Check sheet for the modelled part. Datum: model origin and axes. Units: mm. A direction names the side the tool comes from. Round coordinates to 2 decimals unless told otherwise and drop trailing zeros. Order: outer loops, then holes, each group sorted by start corner. A loop starts at its lowest first (then second) coordinate and runs counter-clockwise, first axis right, second up. Notation, with made-up numbers: (5, -37.5) -> (37, -37.5) arc R22 ccw to (37, -22.5) -> close; hole circle Ø10 at (86, -26). An arc over 180 degrees is marked (long way). Answer in a Markdown table with one row per item.
from build123d import *

# Parameters (mm, degrees)
CUT_EXTRUDE_1_DEPTH = 4
FILLET_1_R          = 0.3
SKETCH_3_R          = 3
CUT_EXTRUDE_2_DEPTH = 25


with BuildPart() as part:
    # Эскиз1 → Повернуть1 (revolve)
    with BuildSketch(Plane.XY, mode=Mode.PRIVATE) as revolve_1_sk:
        with BuildLine():
            Line((0, 157), (0, 0))
            Line((0, 0), (23, 0))
            Line((23, 0), (23, 3.5))
            Line((23, 3.5), (14, 3.5))
            Line((14, 3.5), (14, 5.5))
            Line((14, 5.5), (15, 5.5))
            Line((15, 5.5), (15, 30.5))
            Line((15, 30.5), (13.5, 30.5))
            ThreePointArc((13.5, 30.5), (12.792893219, 30.792893219), (12.5, 31.5))
            Line((12.5, 31.5), (12.5, 123.5))
            Line((12.5, 123.5), (10.5, 125.5))
            Line((10.5, 125.5), (9, 125.5))
            Line((9, 125.5), (9, 127.5))
            Line((9, 127.5), (10, 127.5))
            Line((10, 127.5), (10, 155.5))
            Line((10, 155.5), (8.5, 157))
            Line((8.5, 157), (0, 157))
        make_face()
    revolve(revolve_1_sk.sketch.rotate(Axis((0, 157, 0), (0, -1, 0)), 180), axis=Axis((0, 157, 0), (0, -1, 0)))

    # Эскиз2 → Вырез-Вытянуть1 (cut)
    with BuildSketch(Plane.XY.offset(12.5)):
        with BuildLine():
            Line((5, 45.5), (5, 85.5))
            ThreePointArc((5, 85.5), (0, 90.5), (-5, 85.5))
            Line((-5, 85.5), (-5, 45.5))
            ThreePointArc((-5, 45.5), (0, 40.5), (5, 45.5))
        make_face()
    extrude(amount=-CUT_EXTRUDE_1_DEPTH, mode=Mode.SUBTRACT)

    # Скругление1
    fillet_1_edges = [part.edges().sort_by_distance(p)[0] for p in [
        (0, 40.5, 8.5),
        (-5, 65.5, 8.5),
        (0, 90.5, 8.5),
        (5, 65.5, 8.5),
    ]]
    fillet(fillet_1_edges, radius=FILLET_1_R)

    # Эскиз3 → Вырез-Вытянуть2 (cut)
    with BuildSketch(Plane.XY.offset(10)):
        with Locations((0, 137.5)):
            Circle(SKETCH_3_R)
    extrude(amount=-CUT_EXTRUDE_2_DEPTH, mode=Mode.SUBTRACT)


solid = part.part
Item 1: Depth check by flat-ended pin: P1, Ø12, axis at y = 26.5, z = 8.5, coming from the +X side; P2, Ø1.3, axis at y = 69.5, z = 11, coming from the +X side; P3, Ø10, axis at x = -17.5, z = 13.5, coming from the +Y side. Enter the tip coordinate at first touch or a pass-through.
Result sheet:
| item | result |
|---|---|
| P1 | stops at x = 14.79 |
| P2 | stops at x = 7.01 |
| P3 | stops at y = 3.5 |
Item 2: Cross-section at D-D (z = 19). Record the boundary of the cut face in (x, y).
Result sheet:
| item | result |
|---|---|
| outline | (-12.96, 0) -> (12.96, 0) -> (12.96, 3.5) -> (-12.96, 3.5) -> close |
Item 3: Cross-section at C-C (x = -19.5). Record the boundary of the cut face in (y, z), and give its area (3 significant figures).
Result sheet:
| item | result |
|---|---|
| outline | (0, -12.2) -> (3.5, -12.2) -> (3.5, 12.2) -> (0, 12.2) -> close |
| area | 85.4 mm^2 |
Item 4: Set-up check for faces 1 (the flat face through (0, 157, 0)), 2 (the cylindrical face through (-12.932, 4.514, 5.362)), 3 (the flat face through (5, 65, 10)), 4 (the cylindrical face through (-9.54, 141.7, -3)): record each of +Z, -Z, +X, -X, +Y, -Y from which the full face is reachable in a straight line by a thin tool's end or side.
Result sheet:
| item | result |
|---|---|
| face 1 | +Z, -Z, +X, -X, +Y |
| face 2 | none |
| face 3 | +Z |
| face 4 | +Y |
Item 5: Scan lines: line 1 (Y direction, x = 0, z = -4.5); line 2 (X direction, y = 137.5, z = 0.25); line 3 (Y direction, x = -17, z = 5). Record each from-to range of solid material in increasing order. Write a range as [from, to].
Result sheet:
| item | result |
|---|---|
| line 1 | y = [0, 134.5], [140.5, 157] |
| line 2 | x = [-10, -3], [3, 10] |
| line 3 | y = [0, 3.5] |
Item 6: Cross-section at B-B (y = 137.5). Record the boundary of the cut face in (x, z).
Result sheet:
| item | result |
|---|---|
| outline | (-3, -9.54) -> (-3, 9.54) arc R10 ccw to start; (3, -9.54) arc R10 ccw to (3, 9.54) -> close |
Item 7: Cross-section at A-A (y = 62.5). Record the boundary of the cut face in (x, z), and give its area (3 significant figures).
Result sheet:
| item | result |
|---|---|
| outline | (-5, 8.8) -> (-5, 11.46) arc R12.5 ccw (long way) to (5, 11.46) -> (5, 8.8) arc R0.3 cw to (4.7, 8.5) -> (-4.7, 8.5) arc R0.3 cw to start |
| area | 454 mm^2 |
